```python
from build123d import *

# Parameters (mm, degrees)
SKETCH1_R           = 2.585044133
BOSS_EXTRUDE1_DEPTH = 7.62


with BuildPart() as part:
    # Sketch1 → Boss-Extrude1 (new body)
    with BuildSketch(Plane(origin=(0, 0, 0), x_dir=(1, 0, 0), z_dir=(0, 1, 0))):
        with BuildLine():
            Line((-58.744472787, 21.18875714), (-58.863577215, 32.44818208))
            Line((-58.863577215, 32.44818208), (-73.152298059, 46.437769379))
            Line((-73.152298059, 46.437769379), (-74.797762466, 46.42036333))
            ThreePointArc((-74.797762466, 46.42036333), (-74.712288392, 46.256361266), (-74.638974072, 46.086574622))
            ThreePointArc((-74.638974072, 46.086574622), (-74.738493774, 45.929751081), (-74.84205687, 45.775567815))
            ThreePointArc((-74.84205687, 45.775567815), (-75.79237137, 45.916884294), (-76.622213572, 46.401063925))
            ThreePointArc((-76.622213572, 46.401063925), (-76.899486556, 46.095069224), (-77.199547344, 45.811385265))
            ThreePointArc((-77.199547344, 45.811385265), (-76.697921552, 44.991971107), (-76.536533716, 44.044858674))
            ThreePointArc((-76.536533716, 44.044858674), (-76.688491702, 43.938057155), (-76.843174908, 43.835242273))
            ThreePointArc((-76.843174908, 43.835242273), (-77.667071549, 44.32947129), (-78.248458251, 45.094361803))
            ThreePointArc((-78.248458251, 45.094361803), (-78.621724189, 44.917767339), (-79.00750536, 44.770505828))
            ThreePointArc((-79.00750536, 44.770505828), (-78.857639781, 43.82150198), (-79.070981099, 42.884723736))
            ThreePointArc((-79.070981099, 42.884723736), (-79.252243144, 42.844203803), (-79.434497344, 42.808409938))
            ThreePointArc((-79.434497344, 42.808409938), (-80.00654533, 43.580309605), (-80.250965679, 44.509463354))
            ThreePointArc((-80.250965679, 44.509463354), (-80.663398214, 44.489154033), (-81.076168083, 44.5007342))
            ThreePointArc((-81.076168083, 44.5007342), (-81.300878392, 43.566617894), (-81.856469582, 42.782789835))
            ThreePointArc((-81.856469582, 42.782789835), (-82.039440183, 42.81472028), (-82.221518827, 42.851396724))
            ThreePointArc((-82.221518827, 42.851396724), (-82.454629039, 43.783452315), (-82.32487225, 44.735414064))
            ThreePointArc((-82.32487225, 44.735414064), (-82.713682269, 44.874481796), (-83.090600365, 45.043140665))
            ThreePointArc((-83.090600365, 45.043140665), (-83.655676454, 44.266122641), (-84.468933795, 43.754575485))
            ThreePointArc((-84.468933795, 43.754575485), (-84.625757336, 43.854095187), (-84.779940601, 43.957658283))
            ThreePointArc((-84.779940601, 43.957658283), (-84.638624122, 44.907972782), (-84.154444491, 45.737814985))
            ThreePointArc((-84.154444491, 45.737814985), (-84.460439193, 46.015087969), (-84.744123152, 46.315148756))
            ThreePointArc((-84.744123152, 46.315148756), (-85.563537309, 45.813522965), (-86.510649743, 45.652135128))
            ThreePointArc((-86.510649743, 45.652135128), (-86.617451261, 45.804093115), (-86.720266143, 45.958776321))
            ThreePointArc((-86.720266143, 45.958776321), (-86.226037126, 46.782672961), (-85.461146613, 47.364059664))
            ThreePointArc((-85.461146613, 47.364059664), (-85.637741078, 47.737325602), (-85.785002589, 48.123106773))
            ThreePointArc((-85.785002589, 48.123106773), (-86.734006437, 47.973241194), (-87.670784681, 48.186582511))
            ThreePointArc((-87.670784681, 48.186582511), (-87.711304614, 48.367844557), (-87.747098479, 48.550098756))
            ThreePointArc((-87.747098479, 48.550098756), (-86.975198811, 49.122146743), (-86.046045062, 49.366567091))
            ThreePointArc((-86.046045062, 49.366567091), (-86.066354384, 49.778999627), (-86.054774217, 50.191769496))
            ThreePointArc((-86.054774217, 50.191769496), (-86.988890523, 50.416479804), (-87.772718581, 50.972070995))
            ThreePointArc((-87.772718581, 50.972070995), (-87.740788136, 51.155041596), (-87.704111693, 51.33712024))
            ThreePointArc((-87.704111693, 51.33712024), (-86.772056102, 51.570230452), (-85.820094353, 51.440473663))
            ThreePointArc((-85.820094353, 51.440473663), (-85.681026621, 51.829283682), (-85.512367752, 52.206201778))
            ThreePointArc((-85.512367752, 52.206201778), (-86.289385775, 52.771277867), (-86.800932932, 53.584535208))
            ThreePointArc((-86.800932932, 53.584535208), (-86.701413229, 53.741358749), (-86.597850134, 53.895542014))
            ThreePointArc((-86.597850134, 53.895542014), (-85.647535634, 53.754225535), (-84.817693432, 53.270045904))
            ThreePointArc((-84.817693432, 53.270045904), (-84.540420448, 53.576040606), (-84.24035966, 53.859724565))
            ThreePointArc((-84.24035966, 53.859724565), (-84.741985451, 54.679138722), (-84.903373288, 55.626251155))
            ThreePointArc((-84.903373288, 55.626251155), (-84.751415301, 55.733052674), (-84.596732096, 55.835867556))
            ThreePointArc((-84.596732096, 55.835867556), (-83.772835455, 55.341638539), (-83.191448752, 54.576748026))
            ThreePointArc((-83.191448752, 54.576748026), (-82.818182815, 54.75334249), (-82.432401643, 54.900604001))
            ThreePointArc((-82.432401643, 54.900604001), (-82.582267223, 55.84960785), (-82.368925905, 56.786386093))
            ThreePointArc((-82.368925905, 56.786386093), (-82.18766386, 56.826906026), (-82.00540966, 56.862699892))
            ThreePointArc((-82.00540966, 56.862699892), (-81.433361673, 56.090800224), (-81.188941325, 55.161646475))
            ThreePointArc((-81.188941325, 55.161646475), (-80.77650879, 55.181955796), (-80.363738921, 55.17037563))
            ThreePointArc((-80.363738921, 55.17037563), (-80.139028612, 56.104491936), (-79.583437422, 56.888319994))
            ThreePointArc((-79.583437422, 56.888319994), (-79.400466821, 56.856389549), (-79.218388177, 56.819713106))
            ThreePointArc((-79.218388177, 56.819713106), (-78.985277965, 55.887657515), (-79.115034753, 54.935695766))
            ThreePointArc((-79.115034753, 54.935695766), (-78.726224734, 54.796628034), (-78.349306639, 54.627969164))
            ThreePointArc((-78.349306639, 54.627969164), (-77.78423055, 55.404987188), (-76.970973209, 55.916534344))
            ThreePointArc((-76.970973209, 55.916534344), (-76.814149668, 55.817014642), (-76.659966403, 55.713451547))
            ThreePointArc((-76.659966403, 55.713451547), (-76.801282881, 54.763137047), (-77.285462512, 53.933294844))
            ThreePointArc((-77.285462512, 53.933294844), (-76.979467811, 53.656021861), (-76.695783852, 53.355961073))
            ThreePointArc((-76.695783852, 53.355961073), (-75.876369695, 53.857586864), (-74.929257261, 54.018974701))
            ThreePointArc((-74.929257261, 54.018974701), (-74.822455743, 53.867016714), (-74.71964086, 53.712333509))
            ThreePointArc((-74.71964086, 53.712333509), (-74.789347103, 53.541033964), (-74.871332746, 53.375260478))
            Line((-74.871332746, 53.375260478), (-70.346139099, 53.423128873))
            Line((-70.346139099, 53.423128873), (-50.484046566, 33.9768481))
            Line((-50.484046566, 33.9768481), (-50.373431547, 23.519961391))
            Line((-50.373431547, 23.519961391), (-48.757825737, 19.872187168))
            ThreePointArc((-48.757825737, 19.872187168), (-32.369822631, -18.023926027), (-49.536764273, -55.573601869))
            Line((-49.536764273, -55.573601869), (-57.931525987, -55.662403321))
            ThreePointArc((-57.931525987, -55.662403321), (-40.764719029, -17.050929449), (-58.744472787, 21.18875714))
        make_face()
        with Locations(Location((-80.719953502, 49.835554915, 0), (0, 0, 90))):
            Circle(SKETCH1_R, mode=Mode.SUBTRACT)
    extrude(amount=BOSS_EXTRUDE1_DEPTH)


solid = part.part
```
Work out the finished part from the listing and answer in its coordinate system (mm). A direction names the side the tool comes from. Give positions to 0.01 mm unless a question says otherwise; leave off trailing zeros. Order: outer loops, then holes, each group sorted by start corner. A loop starts at its lowest first (then second) coordinate and runs counter-clockwise, first axis right, second up. Notation, with made-up numbers: M 57,30.25 L 89,30.25 A28 cw 89,65.25 Z; hole C -28,-27 d6. An arc over 180 degrees is marked long. Return JSON: item names as keys, results as strings.
1) For a pull along Z with two mould halves and no side action, classify faces 4 (the cylindrical face through (-32.367, 3.757, 17.429)), 5 (the cylindrical face through (-40.76, 3.76, 17.66)), 6 (the flat face through (-45.6, 7.62, -5)) as +Z half, -Z half, draft (parallel to the pull), parting line (faces both ways), or undercut.
Resolved:
{"face 4": "parting line", "face 5": "undercut", "face 6": "draft"}
2) This flat-tipped pin is pushed along its axis until it touches: pin 1 (4 mm diameter, centred on y = 3.5, z = -18, fed in from -X). Where does it stop, or does it pass through?
Resolved:
{"pin 1": "x = -57.39"}
3) Section A-A, the plane x = -43.5 is taken. Write down the section's boundary in (y, z).
Resolved:
{"outline": "M 0,-14.24 L 7.62,-14.24 L 7.62,1.14 L 0,1.14 Z; M 0,34.04 L 7.62,34.04 L 7.62,49.24 L 0,49.24 Z"}
4) Section B-B, the plane z = -36 is taken. Write down the section's boundary in (x, y), plus the area to 3 significant figures.
Resolved:
{"outline": "M -62.49,0 L -52.55,0 L -52.55,7.62 L -62.49,7.62 Z", "area": "75.7 mm^2"}
5) Section C-C, the plane x = -37.5 is taken. Write down the section's boundary in (y, z), plus the area to 3 significant figures.
Resolved:
{"outline": "M 0,-4.75 L 7.62,-4.75 L 7.62,39.75 L 0,39.75 Z", "area": "339 mm^2"}
6) Straight lines are drawn through the part: line 1 along Z through (x, y) = (-84.5, 3.75); line 2 along Z through (x, y) = (-80.5, 4.5); line 3 along X through (y, z) = (6.5, -44). For each, find the intervals that lie inside material, in ascending order. Write a range as [from, to].
Resolved:
{"line 1": "[-55.8, -54.2], [-53.62, -46.05], [-45.23, -43.77]", "line 2": "[-55.18, -52.41], [-47.26, -44.49]", "line 3": "[-84.78, -83.99], [-82.46, -81.15], [-80.16, -78.86], [-77.2, -76.6], [-70.66, -60.72]"}
7) A tool of negligible diameter and unlimited length cuts with its end or side. For faces 1 (the cylindrical face through (-78.857, 3.757, -43.835)), 2 (the flat face through (-49.577, 3.757, -21.722)), 3 (the flat face through (-65.908, 3.757, -39.345)), from which of +Z, -Z, +X, -X, +Y, -Y can it reach the whole face along a straight path? Write none if from no direction.
Resolved:
{"face 1": "+Y, -Y", "face 2": "-Z, +X, +Y, -Y", "face 3": "+Z, +Y, -Y"}
